```python
from build123d import *

# Parameters (mm, degrees)
F0_R     = 2.5
F1_DEPTH = 450


with BuildPart() as f1:
    # F0 (on Front) → F1 (new body)
    with BuildSketch(Plane.XZ):
        with BuildLine():
            ThreePointArc((-30, -13.2), (-29.472792, -14.472792), (-28.2, -15))
            Line((-28.2, -15), (-19, -15))
            ThreePointArc((-19, -15), (-18.292893, -14.707107), (-18, -14))
            Line((-18, -14), (-18, -12.6))
            ThreePointArc((-18, -12.6), (-18.146447, -12.246447), (-18.5, -12.1))
            Line((-18.5, -12.1), (-24.620101, -12.1))
            ThreePointArc((-24.620101, -12.1), (-25.082041, -11.791342), (-24.973654, -11.246447))
            Line((-24.973654, -11.246447), (-19.559441, -5.832233))
            ThreePointArc((-19.559441, -5.832233), (-18.748382, -5.290301), (-17.791674, -5.1))
            Line((-17.791674, -5.1), (-12.208326, -5.1))
            ThreePointArc((-12.208326, -5.1), (-11.251618, -5.290301), (-10.440559, -5.832233))
            Line((-10.440559, -5.832233), (-5.026346, -11.246447))
            ThreePointArc((-5.026346, -11.246447), (-4.917959, -11.791342), (-5.379899, -12.1))
            Line((-5.379899, -12.1), (-11.5, -12.1))
            ThreePointArc((-11.5, -12.1), (-11.853553, -12.246447), (-12, -12.6))
            Line((-12, -12.6), (-12, -14))
            ThreePointArc((-12, -14), (-11.707107, -14.707107), (-11, -15))
            Line((-11, -15), (0, -15))
            Line((0, -15), (0, -12.1))
            Line((0, -12.1), (-1.627208, -12.1))
            Line((-1.627208, -12.1), (-9.167767, -4.559441))
            ThreePointArc((-9.167767, -4.559441), (-9.709699, -3.748382), (-9.9, -2.791674))
            Line((-9.9, -2.791674), (-9.9, 2.791674))
            ThreePointArc((-9.9, 2.791674), (-9.709699, 3.748382), (-9.167767, 4.559441))
            Line((-9.167767, 4.559441), (-1.627208, 12.1))
            Line((-1.627208, 12.1), (0, 12.1))
            Line((0, 12.1), (0, 15))
            Line((0, 15), (-11, 15))
            ThreePointArc((-11, 15), (-11.707107, 14.707107), (-12, 14))
            Line((-12, 14), (-12, 12.6))
            ThreePointArc((-12, 12.6), (-11.853553, 12.246447), (-11.5, 12.1))
            Line((-11.5, 12.1), (-5.379899, 12.1))
            ThreePointArc((-5.379899, 12.1), (-4.917959, 11.791342), (-5.026346, 11.246447))
            Line((-5.026346, 11.246447), (-10.440559, 5.832233))
            ThreePointArc((-10.440559, 5.832233), (-11.251618, 5.290301), (-12.208326, 5.1))
            Line((-12.208326, 5.1), (-17.791674, 5.1))
            ThreePointArc((-17.791674, 5.1), (-18.748382, 5.290301), (-19.559441, 5.832233))
            Line((-19.559441, 5.832233), (-24.973654, 11.246447))
            ThreePointArc((-24.973654, 11.246447), (-25.082041, 11.791342), (-24.620101, 12.1))
            Line((-24.620101, 12.1), (-18.5, 12.1))
            ThreePointArc((-18.5, 12.1), (-18.146447, 12.246447), (-18, 12.6))
            Line((-18, 12.6), (-18, 14))
            ThreePointArc((-18, 14), (-18.292893, 14.707107), (-19, 15))
            Line((-19, 15), (-28.2, 15))
            ThreePointArc((-28.2, 15), (-29.472792, 14.472792), (-30, 13.2))
            Line((-30, 13.2), (-30, 4))
            ThreePointArc((-30, 4), (-29.707107, 3.292893), (-29, 3))
            Line((-29, 3), (-27.6, 3))
            ThreePointArc((-27.6, 3), (-27.246447, 3.146447), (-27.1, 3.5))
            Line((-27.1, 3.5), (-27.1, 9.620101))
            ThreePointArc((-27.1, 9.620101), (-26.791342, 10.082041), (-26.246447, 9.973654))
            Line((-26.246447, 9.973654), (-20.832233, 4.559441))
            ThreePointArc((-20.832233, 4.559441), (-20.290301, 3.748382), (-20.1, 2.791674))
            Line((-20.1, 2.791674), (-20.1, -2.791674))
            ThreePointArc((-20.1, -2.791674), (-20.290301, -3.748382), (-20.832233, -4.559441))
            Line((-20.832233, -4.559441), (-26.246447, -9.973654))
            ThreePointArc((-26.246447, -9.973654), (-26.791342, -10.082041), (-27.1, -9.620101))
            Line((-27.1, -9.620101), (-27.1, -3.5))
            ThreePointArc((-27.1, -3.5), (-27.246447, -3.146447), (-27.6, -3))
            Line((-27.6, -3), (-29, -3))
            ThreePointArc((-29, -3), (-29.707107, -3.292893), (-30, -4))
            Line((-30, -4), (-30, -13.2))
        make_face()
        with Locations((-15, 0)):
            Circle(F0_R, mode=Mode.SUBTRACT)
    extrude(amount=F1_DEPTH)

    # F2: F1 across plane


with BuildPart() as f1_1:
    add(f1.part)
    add(f1.part.mirror(Plane.YZ))


solid = f1_1.part
```
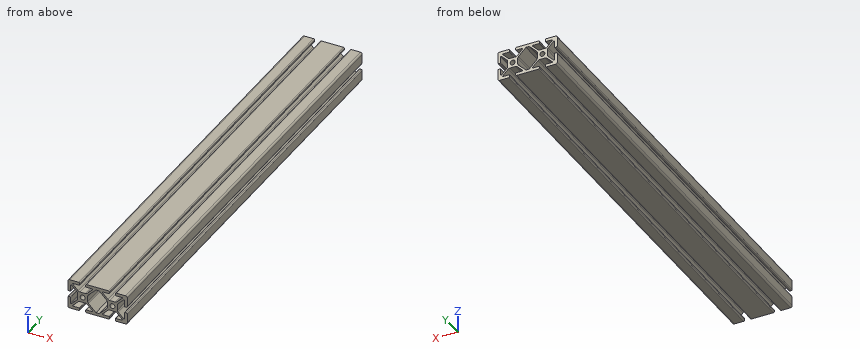
The model under review builds one solid part; all positions refer to its coordinate system, in mm. Give positions to 0.01 mm unless a question says otherwise; leave off trailing zeros. Answer as a JSON object with one key per item and string values.
Q1. To check wall thickness, follow line 1 along Z through (x, y) = (-19.5, -218); line 2 along Z through (x, y) = (9, -351); line 3 along X through (y, z) = (-400, 13). State the ranges of each line that lie inside material, in increasing order.
Worked out:
{"line 1": "z = -15 to -12.1, -5.77 to 5.77, 12.1 to 15", "line 2": "z = -15 to -12.1, -7.27 to -4.73, 4.73 to 7.27, 12.1 to 15", "line 3": "x = -30 to -18, -12 to 12, 18 to 30"}
Q2. Insertion check: pin 1 (3 mm diameter, centred on x = 14.5, y = -256, fed in from -Z); pin 2 (2 mm diameter, centred on x = -22, z = -2.5, fed in from +Y); pin 3 (1.7 mm diameter, centred on y = -303, z = 0.5, fed in from +X). Each pin has a flat end and moves straight along its axis. Give the tip position at first contact, or say it passes through.
Worked out:
{"pin 1": "stops at z = -5.1", "pin 2": "passes through", "pin 3": "stops at x = 20.1"}
Q3. Add section A-A on y = -148. Count the separate pieces of the cut face and the enclosed holes in it, plus the area to 3 significant figures.
Worked out:
{"separate pieces": "1", "enclosed holes": "3", "area": "698 mm^2"}
